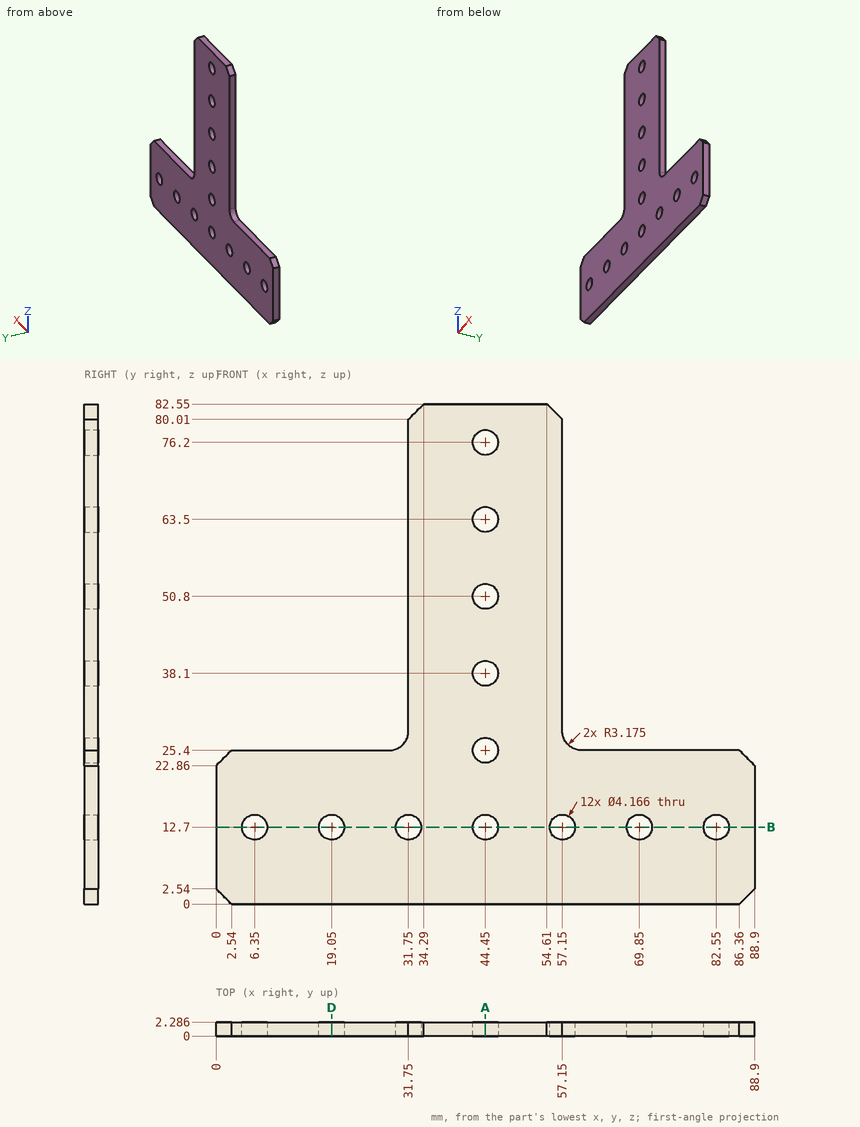
For this review, use the dimensioned drawing (mm, ordinates from the lowest corner) and the shaded views. Give positions to 0.01 mm unless a question says otherwise; leave off trailing zeros. Order: outer loops, then holes, each group sorted by start corner. A loop starts at its lowest first (then second) coordinate and runs counter-clockwise, first axis right, second up. Notation, with made-up numbers: (79, -25) - (110, -25) arc R10 cw to (110, -9) - close; hole circle Ø10 at (-32.5, -9). An arc over 180 degrees is marked (long way). Write item = value, one per line. Start each with the question number.
Q1. Clearance check with flat-ended pins moving along their axes: pin 1 Ø6.5 at (x, z) = (82.55, 12.7) entering from -Y; pin 2 Ø0.7 at (x, y) = (11.5, 1.5) entering from +Z. State where each tip first meets the part, or that it passes through.
Q2. We need section B-B on z = 12.7. State how many separate pieces and enclosed holes the cut face has.
Q3. We need section D-D on x = 19.05. State the section outline as (y, z) points.
Q4. We need section A-A on x = 44.45. State the section outline as (y, z) points.
Q5. To check wall thickness, follow L1, parallel to X at y = 1.8, z = 50.8; L2, parallel to Z at x = 6.35, y = 0.7; L3, parallel to X at y = 1.15, z = 30.5. State the ranges of each line that lie inside material, in increasing order. Write a range as from..to.
Working result:
q1.pin_1 = 0
q1.pin_2 = 25.4
q2.separate_pieces = 8
q2.enclosed_holes = 0
q3.outline = (0, 0) - (2.29, 0) - (2.29, 10.62) - (0, 10.62) - close; (0, 14.78) - (2.29, 14.78) - (2.29, 25.4) - (0, 25.4) - close
q4.outline = (0, 0) - (2.29, 0) - (2.29, 10.62) - (0, 10.62) - close; (0, 14.78) - (2.29, 14.78) - (2.29, 23.32) - (0, 23.32) - close; (0, 27.48) - (2.29, 27.48) - (2.29, 36.02) - (0, 36.02) - close; (0, 40.18) - (2.29, 40.18) - (2.29, 48.72) - (0, 48.72) - close; (0, 52.88) - (2.29, 52.88) - (2.29, 61.42) - (0, 61.42) - close; (0, 65.58) - (2.29, 65.58) - (2.29, 74.12) - (0, 74.12) - close; (0, 78.28) - (2.29, 78.28) - (2.29, 82.55) - (0, 82.55) - close
q5.L1 = 31.75..42.37, 46.53..57.15
q5.L2 = 0..10.62, 14.78..25.4
q5.L3 = 31.75..57.15
